Check sheet for the modelled part. Datum: model origin and axes. Units: mm. A direction names the side the tool comes from. Coordinates: 2 decimals unless noted, no trailing zeros. Use CSV: the item, a comma, the result in double quotes. Start each with the question number.
(1) Scan lines: line 1 (Z direction, x = 25, y = 24); line 2 (X direction, y = -14.5, z = -63) (3 decimals); line 3 (Y direction, x = 4, z = -74.5). Record each from-to range of solid material in increasing order.
(2) Section check A-A on x = -1.5. Give the number of separate pieces and of enclosed holes in the cut face, and give its area (3 significant figures).
(3) Draft check along Z on faces 4 (the flat face through (-25.4, -54, -163)), 5 (the flat face through (0.13, -24.68, 94.26)), 6 (the conical face through (6.946, -35.404, -159.432)). Enter one of: pulls with the +Z half, pulls with the -Z half, needs draft (parallel to the pull), parting line crosses it, or undercut.
(4) Go/stop test with flat-tipped pins: pin 1 Ø10 at (y, z) = (-25, 99) entering from -X (3 decimals); pin 2 Ø4 at (y, z) = (104.5, -131.5) entering from -X; pin 3 Ø2 at (y, z) = (133.5, 93.5) entering from +X. Record where each tip stops, or that it passes through.
(5) Set-up check for faces 1 (the cylindrical face through (0.133, 7.823, 43.756)), 2 (the flat face through (9.525, -74, -62)), 3 (the cylindrical face through (0.089, -21.079, 160.547)): record each of +Z, -Z, +X, -X, +Y, -Y from which the full face is reachable in a straight line by a thin tool's end or side.
from build123d import *

# Parameters (mm, degrees)
CUT_EXTRUDE1_DEPTH = 35.925
CIRPATTERN2_COUNT  = 9
CUT_EXTRUDE2_START = -44.45
SKETCH3_R          = 9.525
CUT_EXTRUDE2_DEPTH = 44.45


with BuildPart() as part:
    # Sketch1 → Revolve2 (revolve)
    with BuildSketch(Plane.XY):
        Polygon((47.625, 9.525), (-25.4, 9.525), (-25.4, 44.45), (-9.525, 44.45), (-9.525, 149.225), (-12.7, 149.225), (-22.225, 171.45), (-25.4, 171.45), (-25.4, 184.15), (-15.875, 184.15), (-6.35, 161.925), (6.35, 161.925), (15.875, 184.15), (25.4, 184.15), (25.4, 171.45), (22.225, 171.45), (12.7, 149.225), (9.525, 149.225), (9.525, 44.45), (47.625, 44.45), align=None)
    revolve(axis=Axis((-229.110116, 0, 0), (1, 0, 0)))

    # Sketch2 → Cut-Extrude1 (cut, through all)
    with BuildSketch(Plane(origin=(9.525, 0, 0), x_dir=(0, 0, -1), z_dir=(1, 0, 0))):
        with BuildLine():
            Line((-7.49963, 43.812761), (-43.506893, 142.741903))
            ThreePointArc((-43.506893, 142.741903), (0, 149.225), (43.506893, 142.741903))
            Line((43.506893, 142.741903), (7.49963, 43.812761))
            ThreePointArc((7.49963, 43.812761), (0, 44.45), (-7.49963, 43.812761))
        make_face()
    cut_extrude1 = extrude(amount=-CUT_EXTRUDE1_DEPTH, mode=Mode.SUBTRACT)

    # CirPattern2: Cut-Extrude1 ×9 about axis
    cirpattern2_axis = Axis((0, 0, 0), (1, 0, 0))
    for i in range(1, CIRPATTERN2_COUNT):
        add(cut_extrude1.rotate(cirpattern2_axis, i * 360 / CIRPATTERN2_COUNT), mode=Mode.SUBTRACT)

    # Sketch3 → Cut-Extrude2 (cut)
    with BuildSketch(Plane(origin=(0, 44.45, 0), x_dir=(1, 0, 0), z_dir=(0, 1, 0)).offset(CUT_EXTRUDE2_START)):
        with Locations((25.4, 0)):
            Circle(SKETCH3_R)
    extrude(amount=CUT_EXTRUDE2_DEPTH, mode=Mode.SUBTRACT)


solid = part.part
Outcome:
1,line 1,"z = -182.58 to -169.76, -37.41 to -9.52, 9.52 to 37.41, 169.76 to 182.58"
1,line 2,"x = -9.525 to 9.525"
1,line 3,"y = -143.77 to -129.3, -101.13 to -76.44, -21.2 to -5.08, 33.85 to 52.18, 129.3 to 143.77"
2,separate pieces,"1"
2,enclosed holes,"10"
2,area,"33,300 mm²"
3,face 4,"needs draft"
3,face 5,"undercut"
3,face 6,"parting line crosses it"
4,pin 1,"stops at x = -9.525"
4,pin 2,"stops at x = -21.59"
4,pin 3,"stops at x = 19.03"
5,face 1,"+X, -X"
5,face 2,"+X"
5,face 3,"none"
